The model under review builds one solid part; all positions refer to its coordinate system, in mm. Face numbers are marked on the shaded views. Coordinates: 2 decimals unless noted, no trailing zeros. Order: outer loops, then holes, each group sorted by start corner. A loop starts at its lowest first (then second) coordinate and runs counter-clockwise, first axis right, second up.
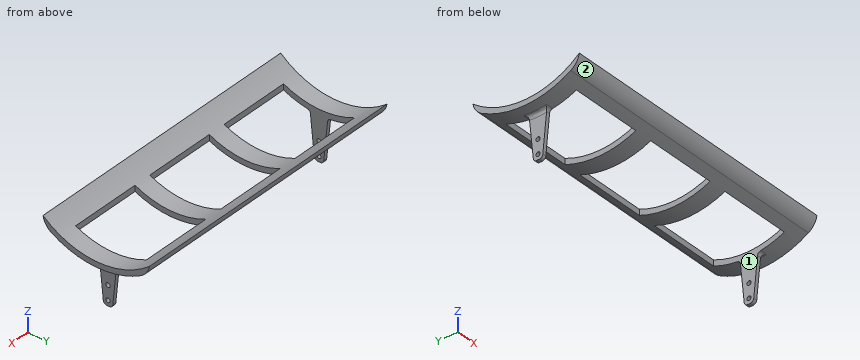
from build123d import *

# Parameters (mm, degrees)
BOSS_EXTRUDE1_DEPTH = 101.6
SKETCH2_W           = 50.8
SKETCH2_H           = 50.8
CUT_EXTRUDE1_DEPTH  = 126.723585695
FILLET1_R           = 12.7
BOSS_EXTRUDE4_START = -2.54
SKETCH6_R           = 1.524
BOSS_EXTRUDE4_DEPTH = 2.54
FILLET4_R           = 2.54


with BuildPart() as part:
    # Sketch1 → Boss-Extrude1 (new, symmetric)
    with BuildSketch(Plane(origin=(0, 0, 0), x_dir=(0, 0, -1), z_dir=(1, 0, 0))):
        with BuildLine():
            Line((50.8, -38.1), (45.948733388, -38.1))
            ThreePointArc((45.948733388, -38.1), (59.69, 0), (45.948733388, 38.1))
            Line((45.948733388, 38.1), (50.8, 38.1))
            ThreePointArc((50.8, 38.1), (63.5, 0), (50.8, -38.1))
        make_face()
    extrude(amount=BOSS_EXTRUDE1_DEPTH, both=True)

    # Sketch2 → Cut-Extrude1 (cut, through all)
    with BuildSketch(Plane.XY):
        with Locations((-63.5, 0)):
            Rectangle(SKETCH2_W, SKETCH2_H)
        with Locations((63.5, 0)):
            Rectangle(SKETCH2_W, SKETCH2_H)
        Rectangle(SKETCH2_W, SKETCH2_H)
    extrude(amount=-CUT_EXTRUDE1_DEPTH, mode=Mode.SUBTRACT)

    # Fillet1
    # the kernel refuses this fillet: 12.7 mm, written as the material it takes off along each edge
    with BuildSketch(Plane(origin=(-120.021720302, 38.1, -50.8), x_dir=(0, -0.8334649822738217, -0.5525722788226877), z_dir=(1, 0, 0))) as fillet1_piece_1:
        with BuildLine():
            CenterArc((6.631819309, -12.678604985), FILLET1_R, 86.673763994, 50.487243594)
            Line((-2.680675447, -4.04336084), (-2.866925342, -3.870655958))
            ThreePointArc((-2.866925342, -3.870655958), (-1.552037829, -1.881327061), (-0.211700105, 0.140353359))
            Line((-0.211700105, 0.140353359), (-0.014737376, 0.2535721))
            ThreePointArc((-0.014737376, 0.2535721), (3.68434406, 0.360975077), (7.383425497, 0.2535721))
            Line((7.383425497, 0.2535721), (7.368688121, 0))
        make_face()
    extrude(amount=240.043440604, mode=Mode.SUBTRACT)
    with BuildSketch(Plane(origin=(-120.021720302, -38.1, -50.8), x_dir=(0, 0, 1), z_dir=(1, 0, 0))) as fillet1_piece_2:
        with BuildLine():
            CenterArc((6.90261377, -12.533234811), FILLET1_R, 99.295330772, 50.487243594)
            Line((-4.071732787, -6.141543514), (-4.291219718, -6.013709688))
            ThreePointArc((-4.291219718, -6.013709688), (-2.33672648, -2.871306936), (-0.2032, 0.1524))
            Line((-0.2032, 0.1524), (0, 0.254))
            ThreePointArc((0, 0.254), (2.425633306, 0.254), (4.810239668, 0.250664696))
            Line((4.810239668, 0.250664696), (4.851266612, 0))
        make_face()
    extrude(amount=240.043440604, mode=Mode.SUBTRACT)

    # Sketch6 → Boss-Extrude4 (add)
    with BuildSketch(Plane.ZY.offset(-88.9).offset(BOSS_EXTRUDE4_START)):
        with BuildLine():
            Line((-63.181702256, -6.35), (-94.931702256, -3.175))
            Line((-94.931702256, -3.175), (-94.931702256, 3.175))
            Line((-94.931702256, 3.175), (-63.181702256, 6.35))
            ThreePointArc((-63.181702256, 6.35), (-63.5, 0), (-63.181702256, -6.35))
        make_face()
        with Locations((-91.121702256, 0)):
            Circle(SKETCH6_R, mode=Mode.SUBTRACT)
        with Locations((-80.961702256, 0)):
            Circle(SKETCH6_R, mode=Mode.SUBTRACT)
    boss_extrude4 = extrude(amount=BOSS_EXTRUDE4_DEPTH)

    # Mirror2: Boss-Extrude4 across plane
    add(boss_extrude4.mirror(Plane(origin=(0, 0, 0), x_dir=(0, 0, 1), z_dir=(1, 0, 0))))

    # Fillet4
    fillet4_edges = [part.edges().sort_by_distance(p)[0] for p in [
        (90.17, 6.35, -63.181702256),
        (90.17, -6.35, -63.181702256),
        (90.17, -3.175, -94.931702256),
        (90.17, 3.175, -94.931702256),
        (-91.44, 0, -63.5),
        (-90.17, -6.35, -63.181702256),
        (-90.17, 6.35, -63.181702256),
        (-90.17, 3.175, -94.931702256),
        (-90.17, -3.175, -94.931702256),
        (91.44, 0, -63.5),
    ]]
    fillet(fillet4_edges, radius=FILLET4_R)


solid = part.part
(1) Consider section B-B (z = -70.5). Give the boundary of the cut face in (x, y), then the cut area to 3 significant figures.
(2) Consider section D-D (y = -17). Give the boundary of the cut face in (x, z).
(3) Consider section C-C (y = 17.5). Give the boundary of the cut face in (x, z), then the cut area to 3 significant figures.
(4) Consider section A-A (x = -0.5). Give the boundary of the cut face in (y, z), then the cut area to 3 significant figures.
(5) The part is to be moulded in two halves that separate along X. For the marked faces 1 and 2, say which applies: +X half, -X half, draft (parallel to the pull), parting line (faces both ways), or undercut.
(6) Insertion check: pin 1 Ø8 at (y, z) = (2.5, -87) entering from -X; pin 2 Ø4.5 at (x, z) = (7, -56) entering from -Y; pin 3 Ø2 at (x, z) = (-53, -55) entering from +Y. Each pin has a flat end and moves straight along its axis. Give the tip position at first contact, or say it passes through.
(7) Wall thickness on line 1 (X direction, y = -19.5, z = -59.5); line 2 (X direction, y = 1, z = -85); line 3 (Z direction, x = -2, y = -27): over which ranges is each line inside the solid? List them lowest first.
Findings:
1. outline: (-91.44, -5.62) - (-88.9, -5.62) - (-88.9, 5.62) - (-91.44, 5.62) - close; (88.9, -5.62) - (91.44, -5.62) - (91.44, 5.62) - (88.9, 5.62) - close
1. area: 57.1 mm2
2. outline: (-101.6, -61.18) - (-88.9, -61.18) - (-88.9, -57.22) - (-101.6, -57.22) - close; (-38.1, -61.18) - (-25.4, -61.18) - (-25.4, -57.22) - (-38.1, -57.22) - close; (25.4, -61.18) - (38.1, -61.18) - (38.1, -57.22) - (25.4, -57.22) - close; (88.9, -61.18) - (101.6, -61.18) - (101.6, -57.22) - (88.9, -57.22) - close
3. outline: (-101.6, -61.04) - (-88.9, -61.04) - (-88.9, -57.07) - (-101.6, -57.07) - close; (-38.1, -61.04) - (-25.4, -61.04) - (-25.4, -57.07) - (-38.1, -57.07) - close; (25.4, -61.04) - (38.1, -61.04) - (38.1, -57.07) - (25.4, -57.07) - close; (88.9, -61.04) - (101.6, -61.04) - (101.6, -57.07) - (88.9, -57.07) - close
3. area: 202 mm2
4. outline: (-38.1, -45.95) arc R12.7 ccw to (-31.96, -54.87) arc R63.5 ccw to (-25.4, -58.2) - (-25.4, -54.02) arc R59.69 cw to start; (25.4, -58.2) arc R63.5 ccw to (31.96, -54.87) arc R12.7 ccw to (38.1, -45.95) arc R59.69 cw to (25.4, -54.02) - close
4. area: 100 mm2
5. face 1: undercut
5. face 2: draft
6. pin 1: stops at x = -91.44
6. pin 2: stops at y = -33.58
6. pin 3: stops at y = 33.26
7. line 1: x = -101.6 to -88.9, -38.1 to -25.4, 25.4 to 38.1, 88.9 to 101.6
7. line 2: x = -91.44 to -88.9, 88.9 to 91.44
7. line 3: z = -57.47 to -53.23
